Geometry check sheet. Reference: the model listing, model coordinates, mm. A direction names the side the tool comes from. Round coordinates to 2 decimals unless told otherwise and drop trailing zeros. Write each loop counter-clockwise with the first axis right and the second up, starting at its lowest first coordinate (ties: lowest second). Pieces come first, ordered by that corner, then holes. Notation, with made-up numbers: M 1.5,53 L 56.5,53 A25 cw 56.5,73 Z; hole C 33,60 d1. An arc over 180 degrees is marked long. Use a Markdown table: item, result.
```python
from build123d import *

# Parameters (mm, degrees)
BOSS_EXTRUDE1_DEPTH = 166


with BuildPart() as part:
    # Sketch1 → Boss-Extrude1 (new body)
    with BuildSketch(Plane.XY):
        with BuildLine():
            Line((-68, 14.557655487), (-66.418275512, 13.549985855))
            Line((-66.418275512, 13.549985855), (-4.216957229, 111.186498042))
            ThreePointArc((-4.216957229, 111.186498042), (0, 113.5), (4.216957229, 111.186498042))
            Line((4.216957229, 111.186498042), (66.418275512, 13.549985855))
            Line((66.418275512, 13.549985855), (68, 14.557655487))
            Line((68, 14.557655487), (68, 37.527193592))
            ThreePointArc((68, 37.527193592), (67.800249272, 38.926338662), (67.216957229, 40.213691634))
            Line((67.216957229, 40.213691634), (16.867828916, 119.245992167))
            ThreePointArc((16.867828916, 119.245992167), (0, 128.5), (-16.867828916, 119.245992167))
            Line((-16.867828916, 119.245992167), (-67.216957229, 40.213691634))
            ThreePointArc((-67.216957229, 40.213691634), (-67.800249272, 38.926338662), (-68, 37.527193592))
            Line((-68, 37.527193592), (-68, 14.557655487))
        make_face()
    extrude(amount=BOSS_EXTRUDE1_DEPTH)


solid = part.part
```
Item 1: Go/stop test with flat-tipped pins: pin 1 (10 mm diameter, centred on x = 35.5, z = 105, fed in from -Y); pin 2 (5 mm diameter, centred on x = 27, y = 74, fed in from -Z); pin 3 (8 mm diameter, centred on x = -50.5, z = 149, fed in from +Y); pin 4 (3 mm diameter, centred on x = 2, z = 120.5, fed in from +Y). Record where each tip stops, or that it passes through.
Outcome:
| item | result |
|---|---|
| pin 1 | stops at y = 54.23 |
| pin 2 | stops at z = 0 |
| pin 3 | stops at y = 72.73 |
| pin 4 | stops at y = 128.49 |
Item 2: Mould release check, pull along X, two halves, no side actions. Record for faces 1 (the face through (0.28, 128.5, 81.84)), 2 (the face through (68, 26, 82)), 3 (the face through (-35.753, 61.685, 81.838)): +X half, -X half, draft (parallel to the pull), parting line (faces both ways), or undercut.
Outcome:
| item | result |
|---|---|
| face 1 | parting line |
| face 2 | +X half |
| face 3 | undercut |
Item 3: Cross-section at C-C, the plane x = -51. Record the cut outline in (y, z).
Outcome:
| item | result |
|---|---|
| outline | M 37.75,0 L 65.67,0 L 65.67,166 L 37.75,166 Z |
Item 4: Cross-section at B-B, the plane z = 118.5. Record the cut outline in (x, y), and give its area (3 significant figures).
Outcome:
| item | result |
|---|---|
| outline | M -68,14.56 L -66.42,13.55 L -4.22,111.19 A5 cw 4.22,111.19 L 66.42,13.55 L 68,14.56 L 68,37.53 A5 ccw 67.22,40.21 L 16.87,119.25 A20 ccw -16.87,119.25 L -67.22,40.21 A5 ccw -68,37.53 Z |
| area | 3,580 mm2 |
Item 5: Material ranges on line 1 along X through (y, z) = (29, 52); line 2 along X through (y, z) = (106, 104); line 3 along X through (y, z) = (121.5, 97.5), recorded low to high. Write a range as from..to.
Outcome:
| item | result |
|---|---|
| line 1 | x = -68..-56.58, 56.58..68 |
| line 2 | x = -25.31..-7.52, 7.52..25.31 |
| line 3 | x = -15.2..15.2 |
Item 6: Access from +Z, -Z, +X, -X, +Y, -Y to the whole of each face (thin tool, end or side, straight path). Record for faces 4 (the face through (42.395, 79.177, 81.838)), 5 (the face through (34.882, 63.052, 81.838)).
Outcome:
| item | result |
|---|---|
| face 4 | +Z, -Z, +X, +Y |
| face 5 | +Z, -Z, -Y |
Item 7: Cross-section at D-D, the plane y = 89. Record the cut outline in (x, z).
Outcome:
| item | result |
|---|---|
| outline | M -36.14,0 L -18.35,0 L -18.35,166 L -36.14,166 Z; M 18.35,0 L 36.14,0 L 36.14,166 L 18.35,166 Z |
Item 8: Cross-section at A-A, the plane y = 28.5. Record the cut outline in (x, z), and give its area (3 significant figures).
Outcome:
| item | result |
|---|---|
| outline | M -68,0 L -56.89,0 L -56.89,166 L -68,166 Z; M 56.89,0 L 68,0 L 68,166 L 56.89,166 Z |
| area | 3,690 mm2 |
